Geometry check sheet. Reference: the model listing, model coordinates, mm. A direction names the side the tool comes from. Give positions to 0.01 mm unless a question says otherwise; leave off trailing zeros. Order: outer loops, then holes, each group sorted by start corner. A loop starts at its lowest first (then second) coordinate and runs counter-clockwise, first axis right, second up. Notation, with made-up numbers: M 70.5,44.5 L 96.5,44.5 A35 ccw 96.5,78.5 Z; hole C 31,-0.75 d3. An arc over 180 degrees is marked long. Answer as CSV lines item,"result".
from build123d import *

# Parameters (mm, degrees)
SKETCH1_W                = 78.232
SKETCH1_H                = 62.23
BOSS_EXTRUDE1_DEPTH      = 128.27
SKETCH2_W                = 43.434
SKETCH2_H                = 88.9
CUT_EXTRUDE1_DEPTH       = 44.45
SKETCH3_W                = 69.342
SKETCH3_H                = 88.9
CUT_EXTRUDE2_DEPTH       = 22.86
CUT_EXTRUDE3_DEPTH       = 163.622297438
CUT_EXTRUDE3_DEPTH_BACK  = 163.622297438
SKETCH4_R                = 3.175
CUT_EXTRUDE4_DEPTH       = 156.317209684
CUT_EXTRUDE4_DEPTH_BACK  = 156.317209684
SKETCH6_R                = 3.4925
CUT_EXTRUDE6_DEPTH       = 163.622297438
CUT_EXTRUDE6_DEPTH_BACK  = 163.622297438
CUT_EXTRUDE7_DEPTH       = 163.622297438
CUT_EXTRUDE7_DEPTH_BACK  = 163.622297438
CUT_EXTRUDE8_DEPTH       = 159.64613082
CUT_EXTRUDE8_DEPTH_BACK  = 107.95
SKETCH9_W                = 44.45
SKETCH9_H                = 5.08
SKETCH10_W               = 38.1
SKETCH10_H               = 80.01
CUT_EXTRUDE9_DEPTH       = 19.05
CUT_EXTRUDE10_START      = -6.35
SKETCH11_W               = 31.75
SKETCH11_H               = 34.29
CUT_EXTRUDE10_DEPTH      = 101.6
CUT_EXTRUDE11_DEPTH      = 159.64613082
CUT_EXTRUDE11_DEPTH_BACK = 159.64613082
SKETCH12_W               = 78.232
SKETCH12_H               = 31.115
BOSS_EXTRUDE4_START      = 4.572
BOSS_EXTRUDE4_DEPTH      = 4.572
CUT_EXTRUDE12_DEPTH      = 151.813823468
CUT_EXTRUDE12_DEPTH_BACK = 5.08
SKETCH18_W               = 16.51
SKETCH18_H               = 3.81
CUT_EXTRUDE13_DEPTH      = 150.066084318
CUT_EXTRUDE13_DEPTH_BACK = 150.066084318
SKETCH19_W               = 88.9
SKETCH19_H               = 12.7
SKETCH13_R               = 4.0005
CUT_EXTRUDE14_DEPTH      = 1.016
MOVE_FACE1_BY            = 0.762
MOVE_FACE1_2_BY          = 0.762
MOVE_FACE1_3_BY          = 0.762
MOVE_FACE1_4_BY          = 0.762


with BuildPart() as part:
    # Sketch1 → Boss-Extrude1 (new body)
    with BuildSketch(Plane.XY):
        with Locations((39.116, 31.115)):
            Rectangle(SKETCH1_W, SKETCH1_H)
    extrude(amount=BOSS_EXTRUDE1_DEPTH)

    # Sketch2 → Cut-Extrude1 (cut)
    with BuildSketch(Plane.XZ):
        with Locations((39.116, 64.135)):
            Rectangle(SKETCH2_W, SKETCH2_H)
    extrude(amount=-CUT_EXTRUDE1_DEPTH, mode=Mode.SUBTRACT)

    # Sketch3 → Cut-Extrude2 (cut)
    with BuildSketch(Plane.XZ):
        with Locations((39.116, 64.135)):
            Rectangle(SKETCH3_W, SKETCH3_H)
    extrude(amount=-CUT_EXTRUDE2_DEPTH, mode=Mode.SUBTRACT)

    # Sketch4 → Cut-Extrude3 (cut, two sides: drawn at the far end of the back side and taken through both)
    with BuildSketch(Plane(origin=(0, 0, 0), x_dir=(-1, 0, 0), z_dir=(0, 0, -1)).offset(-CUT_EXTRUDE3_DEPTH_BACK)):
        with Locations((-39.116, 31.115)):
            Circle(SKETCH4_R)
    extrude(amount=CUT_EXTRUDE3_DEPTH + CUT_EXTRUDE3_DEPTH_BACK, mode=Mode.SUBTRACT)

    # Sketch6 → Cut-Extrude4 (cut, two sides: drawn at the far end of the back side and taken through both)
    with BuildSketch(Plane.XZ.offset(-22.86).offset(-CUT_EXTRUDE4_DEPTH_BACK)):
        with Locations(Location((10.922, 32.893, 0), (0, 0, 270))):
            Circle(SKETCH6_R)
        with Locations(Location((10.922, 44.069, 0), (0, 0, 270))):
            Circle(SKETCH6_R)
        with Locations(Location((10.922, 58.801, 0), (0, 0, 270))):
            Circle(SKETCH6_R)
        with Locations(Location((10.922, 73.025, 0), (0, 0, 270))):
            Circle(SKETCH6_R)
        with Locations(Location((10.922, 84.455, 0), (0, 0, 270))):
            Circle(SKETCH6_R)
        with Locations(Location((10.922, 95.885, 0), (0, 0, 270))):
            Circle(SKETCH6_R)
        with Locations(Location((67.31, 95.885, 0), (0, 0, 270))):
            Circle(SKETCH6_R)
        with Locations(Location((67.31, 84.455, 0), (0, 0, 270))):
            Circle(SKETCH6_R)
        with Locations(Location((67.31, 73.025, 0), (0, 0, 270))):
            Circle(SKETCH6_R)
        with Locations(Location((67.31, 58.801, 0), (0, 0, 270))):
            Circle(SKETCH6_R)
        with Locations(Location((67.31, 44.069, 0), (0, 0, 270))):
            Circle(SKETCH6_R)
        with Locations(Location((67.31, 32.893, 0), (0, 0, 270))):
            Circle(SKETCH6_R)
    extrude(amount=CUT_EXTRUDE4_DEPTH + CUT_EXTRUDE4_DEPTH_BACK, mode=Mode.SUBTRACT)

    # Sketch7 → Cut-Extrude6 (cut, two sides: drawn at the far end of the back side and taken through both)
    with BuildSketch(Plane(origin=(78.232, 0, 0), x_dir=(0, 0, -1), z_dir=(1, 0, 0)).offset(-CUT_EXTRUDE6_DEPTH_BACK)):
        Polygon((-122.936, 58.42), (-122.936, 53.34), (-121.412, 53.34), (-121.412, 10.414), (-122.936, 10.414), (-122.936, 5.334), (-112.776, 5.334), (-112.776, 10.414), (-114.3, 10.414), (-114.3, 53.34), (-112.776, 53.34), (-112.776, 58.42), align=None)
        Polygon((-15.494, 58.42), (-15.494, 53.34), (-13.97, 53.34), (-13.97, 10.414), (-15.494, 10.414), (-15.494, 5.334), (-5.334, 5.334), (-5.334, 10.414), (-6.858, 10.414), (-6.858, 53.34), (-5.334, 53.34), (-5.334, 58.42), align=None)
    extrude(amount=CUT_EXTRUDE6_DEPTH + CUT_EXTRUDE6_DEPTH_BACK, mode=Mode.SUBTRACT)

    # Sketch8 → Cut-Extrude7 (cut, two sides: drawn at the far end of the back side and taken through both)
    with BuildSketch(Plane(origin=(78.232, 0, 0), x_dir=(0, 0, -1), z_dir=(1, 0, 0)).offset(-CUT_EXTRUDE7_DEPTH_BACK)):
        Polygon((-128.27, 62.23), (-125.73, 62.23), (-125.73, 2.54), (-2.54, 2.54), (-2.54, 62.23), (0, 62.23), (0, 0), (-128.27, 0), align=None)
    extrude(amount=CUT_EXTRUDE7_DEPTH + CUT_EXTRUDE7_DEPTH_BACK, mode=Mode.SUBTRACT)

    # Sketch9 → Cut-Extrude8 (cut, two sides: drawn at the far end of the back side and taken through both)
    with BuildSketch(Plane(origin=(0, 0, 2.54), x_dir=(-1, 0, 0), z_dir=(0, 0, -1)).offset(-CUT_EXTRUDE8_DEPTH_BACK)):
        with Locations((-39.116, 57.15)):
            Rectangle(SKETCH9_W, SKETCH9_H)
    extrude(amount=CUT_EXTRUDE8_DEPTH + CUT_EXTRUDE8_DEPTH_BACK, mode=Mode.SUBTRACT)

    # Sketch10 → Cut-Extrude9 (cut)
    with BuildSketch(Plane(origin=(0, 62.23, 0), x_dir=(1, 0, 0), z_dir=(0, 1, 0))):
        with Locations((39.243, -64.135)):
            Rectangle(SKETCH10_W, SKETCH10_H)
    extrude(amount=-CUT_EXTRUDE9_DEPTH, mode=Mode.SUBTRACT)

    # Sketch11 → Cut-Extrude10 (cut)
    with BuildSketch(Plane(origin=(0, 0, 108.585), x_dir=(-1, 0, 0), z_dir=(0, 0, -1)).offset(CUT_EXTRUDE10_START)):
        with Locations((-39.116, 31.115)):
            Rectangle(SKETCH11_W, SKETCH11_H)
    extrude(amount=CUT_EXTRUDE10_DEPTH, mode=Mode.SUBTRACT)

    # Sketch12 → Cut-Extrude11 (cut, two sides: drawn at the far end of the back side and taken through both)
    with BuildSketch(Plane.XY.offset(125.73).offset(-CUT_EXTRUDE11_DEPTH_BACK)):
        with Locations((39.116, 46.6725)):
            Rectangle(SKETCH12_W, SKETCH12_H)
    extrude(amount=CUT_EXTRUDE11_DEPTH + CUT_EXTRUDE11_DEPTH_BACK, mode=Mode.SUBTRACT)

    # Sketch17 → Boss-Extrude4 (add)
    with BuildSketch(Plane(origin=(0, 0, 2.54), x_dir=(-1, 0, 0), z_dir=(0, 0, -1)).offset(BOSS_EXTRUDE4_START)):
        with BuildLine():
            Line((-78.232, 31.115), (-42.291, 31.115))
            ThreePointArc((-42.291, 31.115), (-41.36106403, 28.86993597), (-39.116, 27.94))
            ThreePointArc((-39.116, 27.94), (-36.87093597, 28.86993597), (-35.941, 31.115))
            Line((-35.941, 31.115), (0, 31.115))
            Line((0, 31.115), (0, 2.54))
            Line((0, 2.54), (-78.232, 2.54))
            Line((-78.232, 2.54), (-78.232, 31.115))
        make_face()
    extrude(amount=-BOSS_EXTRUDE4_DEPTH)

    # Sketch18 → Cut-Extrude12 (cut, two sides: drawn at the far end of the back side and taken through both)
    with BuildSketch(Plane(origin=(0, 31.115, 0), x_dir=(1, 0, 0), z_dir=(0, 1, 0)).offset(-CUT_EXTRUDE12_DEPTH_BACK)):
        with Locations((39.116, -2.413)):
            Rectangle(SKETCH18_W, SKETCH18_H)
    extrude(amount=CUT_EXTRUDE12_DEPTH + CUT_EXTRUDE12_DEPTH_BACK, mode=Mode.SUBTRACT)

    # Sketch19 → Cut-Extrude13 (cut, two sides: drawn at the far end of the back side and taken through both)
    with BuildSketch(Plane.ZY.offset(-73.787).offset(-CUT_EXTRUDE13_DEPTH_BACK)):
        with Locations((64.248626707, 8.89)):
            Rectangle(SKETCH19_W, SKETCH19_H)
    extrude(amount=CUT_EXTRUDE13_DEPTH + CUT_EXTRUDE13_DEPTH_BACK, mode=Mode.SUBTRACT)

    # Sketch13 → Cut-Extrude14 (cut)
    with BuildSketch(Plane(origin=(0, 31.115, 0), x_dir=(1, 0, 0), z_dir=(0, 1, 0))):
        with Locations(Location((69.342, -20.32, 0), (0, 0, 270))):
            Circle(SKETCH13_R)
        with Locations(Location((8.89, -107.95, 0), (0, 0, 270))):
            Circle(SKETCH13_R)
    extrude(amount=-CUT_EXTRUDE14_DEPTH, mode=Mode.SUBTRACT)

    # Move Face1: a face moved inward by 0.762
    extrude(part.faces().sort_by_distance((39.116, 20.675603328, 6.858))[0], amount=MOVE_FACE1_BY, dir=(0, 0, -1), mode=Mode.SUBTRACT)

    # Move Face1 2: a face moved inward by 0.762
    extrude(part.faces().sort_by_distance((58.674, 20.7645, 13.97))[0], amount=MOVE_FACE1_2_BY, dir=(0, 0, 1), mode=Mode.SUBTRACT)

    # Move Face1 3: a face moved inward by 0.762
    extrude(part.faces().sort_by_distance((58.674, 20.7645, 114.3))[0], amount=MOVE_FACE1_3_BY, dir=(0, 0, -1), mode=Mode.SUBTRACT)

    # Move Face1 4: a face moved inward by 0.762
    extrude(part.faces().sort_by_distance((39.116, 20.675603328, 121.412))[0], amount=MOVE_FACE1_4_BY, dir=(0, 0, 1), mode=Mode.SUBTRACT)


solid = part.part
(1) Section check D-D on x = 16. Enter the section's corners in (y, z) (3 decimals), then the cut area to 3 significant figures.
The answers:
outline,"M 2.54,-2.032 L 31.115,-2.032 L 31.115,6.096 L 10.414,6.096 L 10.414,5.334 L 5.334,5.334 L 5.334,15.494 L 10.414,15.494 L 10.414,14.732 L 31.115,14.732 L 31.115,113.538 L 10.414,113.538 L 10.414,112.776 L 5.334,112.776 L 5.334,122.936 L 10.414,122.936 L 10.414,122.174 L 31.115,122.174 L 31.115,125.73 L 2.54,125.73 L 2.54,108.699 L 15.24,108.699 L 15.24,108.585 L 22.86,108.585 L 22.86,19.685 L 2.54,19.685 Z"
area,"1,380 mm2"
(2) Section check C-C on y = 19.5. Enter the section's corners in (x, z) (3 decimals), then the cut area to 3 significant figures.
The answers:
outline,"M 0,-2.032 L 78.232,-2.032 L 78.232,6.096 L 0,6.096 Z; M 0,14.732 L 23.241,14.732 L 23.241,19.685 L 4.445,19.685 L 4.445,108.585 L 23.241,108.585 L 23.241,113.538 L 0,113.538 Z; M 0,122.174 L 78.232,122.174 L 78.232,125.73 L 0,125.73 Z; M 54.991,14.732 L 78.232,14.732 L 78.232,113.538 L 54.991,113.538 L 54.991,108.585 L 73.787,108.585 L 73.787,19.685 L 54.991,19.685 Z"
area,"2,160 mm2"
(3) Section check B-B on z = 65. Enter the section's corners in (x, y) (3 decimals).
The answers:
outline,"M 0,15.24 L 4.445,15.24 L 4.445,22.86 L 17.399,22.86 L 17.399,31.115 L 0,31.115 Z; M 60.833,22.86 L 73.787,22.86 L 73.787,15.24 L 78.232,15.24 L 78.232,31.115 L 60.833,31.115 Z"
(4) Tool access check on faces 3 (the face through (40, 9, 108.699)), 4 (the face through (39, 26.035, 2)), 5 (the face through (39, 21, 122.174)). Record the directions out of +Z, -Z, +X, -X, +Y, -Y that give a thin tool (end or side, any length) a straight path to the whole face; none if there is none.
The answers:
face 3,"+X, -X, -Y"
face 4,"+Y"
face 5,"+X, -X, +Y"
(5) Draft check along Z on faces 1 (the face through (39.19, 27.94, 5.22)), 2 (the face through (11.076, 27.045, 87.944)). Enter one of: +Z half, -Z half, draft (parallel to the pull), parting line (faces both ways), or undercut.
The answers:
face 1,"draft"
face 2,"undercut"
(6) Material ranges on line 1 (Z direction, x = 5.5, y = 21.5) (3 decimals); line 2 (Z direction, x = 59, y = 13.5) (3 decimals); line 3 (Z direction, x = 72.5, y = 25.25), recorded low to high.
The answers:
line 1,"z = -2.032 to 6.096, 14.732 to 19.685, 108.585 to 113.538, 122.174 to 125.73"
line 2,"z = -2.032 to 6.096, 14.732 to 19.685, 108.699 to 113.538, 122.174 to 125.73"
line 3,"z = -2.03 to 6.1, 14.73 to 113.54, 122.17 to 125.73"
(7) Section check A-A on x = 51. Enter the section's corners in (y, z) (3 decimals).
The answers:
outline,"M 2.54,-2.032 L 31.115,-2.032 L 31.115,6.096 L 10.414,6.096 L 10.414,5.334 L 5.334,5.334 L 5.334,15.494 L 10.414,15.494 L 10.414,14.732 L 13.97,14.732 L 13.97,19.685 L 2.54,19.685 Z; M 2.54,108.699 L 13.97,108.699 L 13.97,113.538 L 10.414,113.538 L 10.414,112.776 L 5.334,112.776 L 5.334,122.936 L 10.414,122.936 L 10.414,122.174 L 31.115,122.174 L 31.115,125.73 L 2.54,125.73 Z"
(8) Gauge pin test, flat ends, axial feed: P1, Ø2.5, axis at x = 7, z = 107, coming from the +Y side; P2, Ø6.5, axis at x = 65, z = 82, coming from the -Y side; P3, Ø11, axis at x = 38.5, z = 12.5, coming from the +Y side. Record the tip position at first contact, or that the pin passes through.
The answers:
P1,"stops at y = 30.1"
P2,"stops at y = 22.86"
P3,"stops at y = 13.97"
